Source: CAD feature listing. Evaluate the final solid. Frame: model axes, mm. A direction names the side the tool comes from. Give positions to 0.01 mm unless a question says otherwise; leave off trailing zeros. Order: outer loops, then holes, each group sorted by start corner. A loop starts at its lowest first (then second) coordinate and runs counter-clockwise, first axis right, second up. Notation, with made-up numbers: M 46.5,31 L 72.5,31 A14 ccw 72.5,43 Z; hole C -33.75,57.25 d9. An arc over 180 degrees is marked long. Answer in a Markdown table with one row per item. Add a question column.
(1) Section query A-A, the plane y = 4. Return loops of the section in (x, z), plus the area to 3 significant figures.
(2) Set-up query: faces 4 (the face through (1, 1.3, -21.1)), 5 (the face through (7, 1, 17)), 6 (the face through (17, 7, 5)), 7 (the face through (14, 21, -13)). Return all of +Z, -Z, +X, -X, +Y, -Y with unobstructed straight access to the full face (end or side cutting, diameter ignored); none if empty.
(3) Mould query, pull axis Y, two halves, no side actions, for faces 1 (the face through (3, 4, 25)), 2 (the face through (3, 10.5, 16)), 3 (the face through (17, 17.5, 0)). Classes: pulls with the +Y half, pulls with the -Y half, needs draft (parallel to the pull), parting line crosses it, or undercut.
(4) Material intervals for line 1 along Z through (x, y) = (15, 2.5); line 2 along X through (y, z) = (7.5, -7.7); line 3 along Y through (x, z) = (20, 8.65), sorted ascending.
(5) Pin query (flat end, axial travel): P1, Ø10, axis at x = 21.5, y = 9, coming from the -Z side; P2, Ø3.5, axis at x = 2.5, z = 16.5, coming from the +Y side; P3, Ø2.5, axis at x = 13.5, z = -12, coming from the -Y side. Return the tip coordinate at first contact, or that it passes through.
(6) Section query B-B, the plane z = -17.5. Return loops of the section in (x, y).
(7) Section query D-D, the plane z = 9. Return loops of the section in (x, y), plus the area to 3 significant figures.
(8) Section query C-C, the plane x = 20. Return loops of the section in (y, z), plus the area to 3 significant figures.
Autodesk Inventor part; units mm, degrees
ref_plane "YZ Plane" through (0, 0, 0) normal (1, 0, 0) x (0, 1, 0)
ref_plane "XZ Plane" through (0, 0, 0) normal (0, 1, 0) x (-1, 0, 0)
ref_plane "XY Plane" through (0, 0, 0) normal (0, 0, 1) x (1, 0, 0)
sketch "Sketch7" plane through (0, 0, 0) normal (1, 0, 0) x (0, 0, -1)
  line L0 (10, -2.5) -> (-10, -2.5)
  line L1 (-10, -2.5) -> (-10, 22.5)
  line L2 (-10, 22.5) -> (10, 22.5)
  line L3 (10, 22.5) -> (10, -2.5)
  line L4 (13, 19.5) -> (10, 19.5)
  line L5 (10, 19.5) -> (10, 22.5)
  line L6 (10, 22.5) -> (13, 22.5)
  line L7 (13, 22.5) -> (13, 19.5)
  line L8 (-10, 19.5) -> (-13, 19.5)
  line L9 (-13, 19.5) -> (-13, 22.5)
  line L10 (-13, 22.5) -> (-10, 22.5)
  line L11 (-10, 22.5) -> (-10, 19.5)
  point P0 (0, -2.5)
  point P1 (0, 22.5)
  dimension "d26" = 20
  dimension "d27" = 25
  dimension "d30" = 3
  dimension "d31" = 3
  dimension "d32" = 3
  dimension "d33" = 3
  dimension "d72" = 0
extrude "Extrusion4" add sketch "Sketch7" along normal blind 28
sketch "Sketch15" plane through (0, -2.5, -10) normal (0, 0, -1) x (-1, 0, 0)
  line L0 (0, 0) -> (-28, 0)
  line L1 (-28, 0) -> (-28, 22)
  point P0 (0, 2.5)
  point P1 (-20, 10)
  dimension "d78" = 8
  dimension "d98" = 10
sketch "Sketch14" plane through (0, -2.5, -10) normal (0, -1, 0) x (1, 0, 0)
  line L0 (7, 15) -> (28, 15)
  line L1 (28, 15) -> (28, 5)
  line L2 (28, 5) -> (7, 5)
  line L3 (7, 5) -> (7, 15)
  line L4 (28, 20) -> (28, 0)
  point P0 (0, 10)
  point P1 (28, 10)
  point P2 (28, 10)
  dimension "d73" = 10
  dimension "d74" = 21
extrude "Extrusion8" cut sketch "Sketch14" against normal blind 20
hole "Hole6" at (20, 7.5, -10) direction (0, 0, 1) diameter 4.134 end through all
sketch "Sketch16" plane through (0, 0, 0) normal (-1, 0, 0) x (0, 0, 1)
  line L0 (25, -2.5) -> (-25, -2.5)
  line L1 (-25, -2.5) -> (-25, 10.5)
  line L2 (-25, 10.5) -> (25, 10.5)
  line L3 (25, 10.5) -> (25, -2.5)
  line L4 (10, -2.5) -> (-10, -2.5)
  line L5 (-10, -2.5) -> (-10, 19.5)
  line L6 (10, 19.5) -> (10, -2.5)
  circle A0 centre (17.5, 4) radius 2.5
  circle A1 centre (-17.5, 4) radius 2.5
  point P0 (0, 0)
  point P1 (25, 4)
  point P2 (-10, -2.5)
  point P3 (-10, 10.5)
  point P4 (10, 10.5)
  point P5 (10, -2.5)
  dimension "d86" = 15
  dimension "d88" = 15
  dimension "d89" = 13
  dimension "d90" = 5
  dimension "d91" = 7.5
  dimension "d92" = 7.5
extrude "Extrusion9" add sketch "Sketch16" against normal blind 7 contours L0 L6 L2 L3 | L0 L1 L2 L5
fillet "Fillet1" radius 2 4 edges at (3.5, -2.5, -25) (3.5, 10.5, -25) (3.5, -2.5, 25) (3.5, 10.5, 25)
sketch "Sketch17" plane through (0, 0, 0) normal (-1, 0, 0) x (0, 0, 1)
  circle A0 centre (17.5, 4) radius 4.5
  circle A1 centre (-17.5, 4) radius 4.5
  circle A2 centre (-17.5, 4) radius 2.5
  circle A3 centre (17.5, 4) radius 2.5
  point P0 (0, 0)
  dimension "d99" = 9
extrude "Extrusion10" cut sketch "Sketch17" against normal blind 2
equation "\"d88\" = d86"
equation "\"d91\" = 0.5 * d88"
equation "\"d92\" = d91"
properties part number "10-03-025"
Values follow:
| question | item | result |
|---|---|---|
| 1 | outline | M 0,-25 L 7,-25 L 7,-20 L 2,-20 L 2,-22 L 0,-22 Z; M 0,-13 L 2,-13 L 2,-15 L 7,-15 L 7,-10 L 28,-10 L 28,-5 L 7,-5 L 7,5 L 28,5 L 28,10 L 7,10 L 7,15 L 2,15 L 2,13 L 0,13 Z; M 0,22 L 2,22 L 2,20 L 7,20 L 7,25 L 0,25 Z |
| 1 | area | 474 mm² |
| 2 | face 4 | -X |
| 2 | face 5 | +Z, +X, -Y |
| 2 | face 6 | +X, -Y |
| 2 | face 7 | -Z, +X, -X, +Y |
| 3 | face 1 | needs draft |
| 3 | face 2 | undercut |
| 3 | face 3 | pulls with the -Y half |
| 4 | line 1 | z = -10 to -5, 5 to 10 |
| 4 | line 2 | x = 0 to 17.93, 22.07 to 28 |
| 4 | line 3 | y = -2.5 to 5.43, 9.57 to 22.5 |
| 5 | P1 | stops at z = -10 |
| 5 | P2 | stops at y = 10.5 |
| 5 | P3 | stops at y = 19.5 |
| 6 | outline | M 0,-2.5 L 7,-2.5 L 7,1.5 L 2,1.5 L 2,-0.5 L 0,-0.5 Z; M 0,8.5 L 2,8.5 L 2,6.5 L 7,6.5 L 7,10.5 L 0,10.5 Z |
| 7 | outline | M 0,-2.5 L 28,-2.5 L 28,22.5 L 0,22.5 Z; hole C 20,7.5 d4.13 |
| 7 | area | 687 mm² |
| 8 | outline | M -2.5,-10 L 5.43,-10 L 5.43,-5 L -2.5,-5 Z; M -2.5,5 L 5.43,5 L 5.43,10 L -2.5,10 Z; M 9.57,-10 L 19.5,-10 L 19.5,-13 L 22.5,-13 L 22.5,13 L 19.5,13 L 19.5,10 L 9.57,10 L 9.57,5 L 17.5,5 L 17.5,-5 L 9.57,-5 Z |
| 8 | area | 277 mm² |
